from build123d import *

# Parameters (mm, degrees)
CUT_EXTRUDE1_DEPTH       = 61.261789517
CUT_EXTRUDE1_DEPTH_BACK  = 61.261789517
SKETCH2_R                = 3
BOSS_EXTRUDE1_REACH      = 83.135
BOSS_EXTRUDE1_END_RADIUS = 25.86032094
SKETCH3_R                = 4
SKETCH3_R_2              = 3


with BuildPart() as part:
    # Sketch1 → Revolve1 (revolve)
    with BuildSketch(Plane.XY, mode=Mode.PRIVATE) as revolve1_sk:
        Polygon((-32, 20.352725591), (32, 20.352725591), (32, 36.352725591), (23, 36.352725591), (23, 28.352725591), (14, 28.352725591), (14, 26.352725591), (-14, 26.352725591), (-14, 28.352725591), (-23, 28.352725591), (-23, 36.352725591), (-32, 36.352725591), align=None)
    revolve(revolve1_sk.sketch.rotate(Axis((-45.635800038, 0.492404651, 0), (1, 0, 0)), 90), axis=Axis((-45.635800038, 0.492404651, 0), (1, 0, 0)))

    # Sketch2 → Cut-Extrude1 (cut, two sides: drawn at the far end of the back side and taken through both)
    with BuildSketch(Plane(origin=(0, 0, 0), x_dir=(1, 0, 0), z_dir=(0, 1, 0)).offset(-CUT_EXTRUDE1_DEPTH_BACK)):
        with Locations(Location((0, 0, 0), (0, 0, 270))):
            Circle(SKETCH2_R)
    extrude(amount=CUT_EXTRUDE1_DEPTH + CUT_EXTRUDE1_DEPTH_BACK, mode=Mode.SUBTRACT)

    # Boss-Extrude1: up to this cylinder (the profile starts outside it)
    boss_extrude1_end = Plane(origin=(0, 0.492404651, 0), z_dir=(-1, 0, 0)) * Cylinder(BOSS_EXTRUDE1_END_RADIUS, 218.99064188, mode=Mode.PRIVATE)
    # Sketch3 → Boss-Extrude1 (add, up to the surface)
    with BuildSketch(Plane(origin=(0, 30, 0), x_dir=(1, 0, 0), z_dir=(0, 1, 0)), mode=Mode.PRIVATE) as boss_extrude1_sk1:
        with Locations(Location((0, 0, 0), (0, 0, 270))):
            Circle(SKETCH3_R)
        with Locations(Location((0, 0, 0), (0, 0, 270))):
            Circle(SKETCH3_R_2, mode=Mode.SUBTRACT)
    boss_extrude1_tool1 = extrude(boss_extrude1_sk1.sketch, amount=-BOSS_EXTRUDE1_REACH, mode=Mode.PRIVATE) - boss_extrude1_end
    add(boss_extrude1_tool1.solids().sort_by_distance((0, 30, -3.886863))[0])


solid = part.part
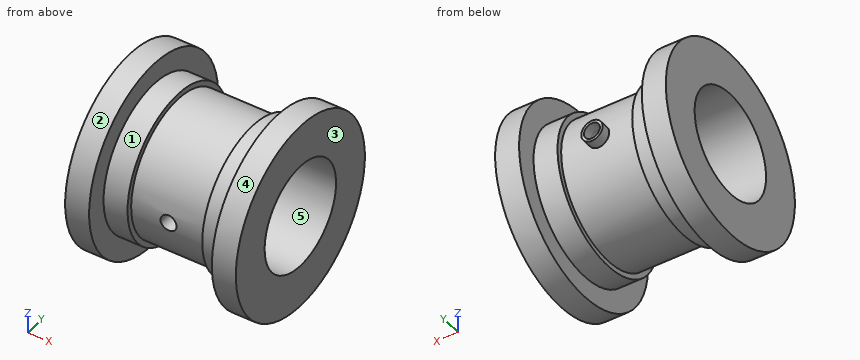
Input: part model. Units: mm. Frame: model coordinates. Face numbers are marked on the shaded views. A direction names the side the tool comes from. Give positions to 0.01 mm unless a question says otherwise; leave off trailing zeros. Loops run counter-clockwise (first coordinate to the right, second up) from the corner with the lowest first, then second, coordinate; pieces in that order, holes last. Notation, with made-up numbers: M 24,9.5 L 68,9.5 A24 ccw 68,40.5 Z; hole C 40.25,44.25 d10. An arc over 180 degrees is marked long. Use CSV: the item, a comma, the result in double quotes.
(1) Section D-D, the plane z = 0. Count the separate pieces of the cut face and the enclosed holes in it, plus the area to 3 significant figures.
Outcome:
separate pieces,"4"
enclosed holes,"0"
area,"1,140 mm²"
(2) Material intervals for L1, parallel to X at y = -23.75, z = 0; L2, parallel to Y at x = -17.5, z = 0; L3, parallel to X at y = 15, z = -26, sorted ascending. Write a range as [from, to].
Outcome:
L1,"x = [-32, -3], [3, 32]"
L2,"y = [-27.37, -19.37], [20.35, 28.35]"
L3,"x = [-32, -23], [23, 32]"
(3) Section B-B, the plane y = -13. Return loops of the section in (x, z).
Outcome:
outline,"M -32,-33.23 L -23,-33.23 L -23,-24.38 L -14,-24.38 L -14,-22.06 L 14,-22.06 L 14,-24.38 L 23,-24.38 L 23,-33.23 L 32,-33.23 L 32,-14.57 L -32,-14.57 Z; M -32,14.57 L 32,14.57 L 32,33.23 L 23,33.23 L 23,24.38 L 14,24.38 L 14,22.06 L -14,22.06 L -14,24.38 L -23,24.38 L -23,33.23 L -32,33.23 Z"
(4) Section A-A, the plane z = -11. Return loops of the section in (x, y).
Outcome:
outline,"M -32,-33.64 L -23,-33.64 L -23,-25.1 L -14,-25.1 L -14,-22.91 L 14,-22.91 L 14,-25.1 L 23,-25.1 L 23,-33.64 L 32,-33.64 L 32,-16.04 L -32,-16.04 Z; M -32,17.03 L 32,17.03 L 32,34.62 L 23,34.62 L 23,26.09 L 14,26.09 L 14,23.9 L -14,23.9 L -14,26.09 L -23,26.09 L -23,34.62 L -32,34.62 Z"
(5) Set-up query: the marked faces 1 and 2. Return all of +Z, -Z, +X, -X, +Y, -Y with unobstructed straight access to the full face (end or side cutting, diameter ignored); none if empty.
Outcome:
face 1,"none"
face 2,"+X, -X"
(6) Pin query (flat end, axial travel): P1, Ø5, axis at x = 0, z = 0, coming from the -Y side; P2, Ø1.5, axis at x = -11.5, z = -16, coming from the +Y side; P3, Ø10, axis at x = 0, z = 2.5, coming from the +Y side; P4, Ø8, axis at x = -22.5, z = -9, coming from the -Y side. Return the tip coordinate at first contact, or that it passes through.
Outcome:
P1,"passes through"
P2,"stops at y = 21.38"
P3,"stops at y = 30"
P4,"stops at y = -35.01"
(7) Section C-C, the plane x = 0. Return loops of the section in (y, z), plus the area to 3 significant figures.
Outcome:
outline,"M -25.19,-3 A25.86 ccw 26.04,-4 L 30,-4 L 30,-3 L 20.12,-3 A19.86 cw -19.14,-3 Z; M -25.19,3 L -19.14,3 A19.86 cw 20.12,3 L 30,3 L 30,4 L 26.04,4 A25.86 ccw Z"
area,"797 mm²"
(8) Pull-direction query (Z, two-part tool) for the marked faces 3, 4 and 5; classes: pulls with the +Z half, pulls with the -Z half, needs draft (parallel to the pull), parting line crosses it, or undercut.
Outcome:
face 3,"needs draft"
face 4,"parting line crosses it"
face 5,"undercut"
